Design review of the part built by this model. Coordinates are the model's own, in mm. Give positions to 0.01 mm unless a question says otherwise; leave off trailing zeros. Order: outer loops, then holes, each group sorted by start corner. A loop starts at its lowest first (then second) coordinate and runs counter-clockwise, first axis right, second up.
```python
from build123d import *

# Parameters (mm, degrees)
SKETCH1_R           = 25
SKETCH1_R_2         = 0.85
BOSS_EXTRUDE1_DEPTH = 1.5875
CUT_EXTRUDE1_REACH  = 5.175
SKETCH2_W           = 3.873993702
SKETCH2_H           = 19.044786736


with BuildPart() as part:
    # Sketch1 → Boss-Extrude1 (new body, symmetric)
    with BuildSketch(Plane.XY):
        Circle(SKETCH1_R)
        Circle(SKETCH1_R_2, mode=Mode.SUBTRACT)
    extrude(amount=BOSS_EXTRUDE1_DEPTH, both=True)

    # Sketch2 → Cut-Extrude1 (cut, up to next)
    with BuildSketch(Plane(origin=(0, 0, -1.5875), x_dir=(-1, 0, 0), z_dir=(0, 0, -1)), mode=Mode.PRIVATE) as cut_extrude1_sk1:
        with Locations((0, 24.522393368)):
            Rectangle(SKETCH2_W, SKETCH2_H)
    cut_extrude1_tool1 = extrude(cut_extrude1_sk1.sketch, amount=-CUT_EXTRUDE1_REACH, mode=Mode.PRIVATE) & part.part
    add(cut_extrude1_tool1.solids().sort_by_distance((0, 24.522393, -1.5875))[0], mode=Mode.SUBTRACT)


solid = part.part
```
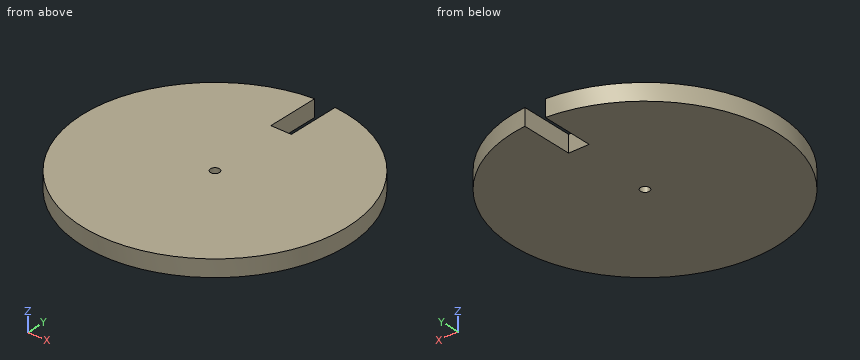
1. Take a section at A-A (y = 0). State the section outline as (x, z) points, then the cut area to 3 significant figures.
Recorded:
outline: (-25, -1.59) - (-0.85, -1.59) - (-0.85, 1.59) - (-25, 1.59) - close; (0.85, -1.59) - (25, -1.59) - (25, 1.59) - (0.85, 1.59) - close
area: 153 mm2
2. Take a section at D-D (y = -18). State the section outline as (x, z) points, then the cut area to 3 significant figures.
Recorded:
outline: (-17.35, -1.59) - (17.35, -1.59) - (17.35, 1.59) - (-17.35, 1.59) - close
area: 110 mm2
3. For pin 1 (1.5 mm diameter, centred on x = 0, y = 0, fed in from -Z); pin 2 (1.6 mm diameter, centred on y = 18.5, z = 0, fed in from +X); pin 3 (1 mm diameter, centred on y = 20, z = 0, fed in from -X), all flat-tipped, find the tip position at first contact; note any pin that passes through.
Recorded:
pin 1: passes through
pin 2: stops at x = 17.66
pin 3: stops at x = -15.64
4. Take a section at C-C (x = 0). State the section outline as (y, z) points.
Recorded:
outline: (-25, -1.59) - (-0.85, -1.59) - (-0.85, 1.59) - (-25, 1.59) - close; (0.85, -1.59) - (15, -1.59) - (15, 1.59) - (0.85, 1.59) - close
5. For line 1 along Y through (x, z) = (0, -0.45); line 2 along X through (y, z) = (15.5, 0.95); line 3 along X through (y, z) = (-10.5, -0.9), list the stretches that pass through material, from the lowest coordinate up.
Recorded:
line 1: y = -25 to -0.85, 0.85 to 15
line 2: x = -19.62 to -1.94, 1.94 to 19.62
line 3: x = -22.69 to 22.69
6. Take a section at B-B (z = 1.05). State the section outline as (x, y) points.
Recorded:
outline: (-1.94, 15) - (-1.94, 24.92) arc R25 ccw (long way) to (1.94, 24.92) - (1.94, 15) - close; hole circle Ø1.7 at (0, 0)
